Can you work these out from the model? Positions are in its coordinate system, mm. Give positions to 0.01 mm unless a question says otherwise; leave off trailing zeros. Loops run counter-clockwise (first coordinate to the right, second up) from the corner with the lowest first, then second, coordinate; pieces in that order, holes last.
Autodesk Inventor part; units mm, degrees
ref_plane "4DUMMY_XY" through (0, 0, 0) normal (1, 0, 0) x (0, 0, -1)
ref_plane "4DUMMY_YZ" through (0, 0, 0) normal (0, 0, -1) x (0, 1, 0)
ref_plane "4DUMMY_ZX" through (0, 0, 0) normal (0, 1, 0) x (1, 0, 0)
sketch "Sketch_15" plane through (-20, 0, 0) normal (1, 0, 0) x (0, 0, -1)
  line L0 (-7.5, 0.85) -> (-6.65, 0)
  line L1 (-6.65, 0) -> (6.65, 0)
  line L2 (6.65, 0) -> (7.5, 0.85)
  line L3 (7.5, 0.85) -> (7.5, 4.768)
  line L4 (7.5, 4.768) -> (5.4163, 5.9696)
  arc A0 (5.1599, 6.9262) -> (5.4163, 5.9696) centre (5.766, 6.576) ccw
  line L5 (5.1599, 6.9262) -> (6.6573, 9.518)
  arc A1 (7.5, 10.8638) -> (6.6573, 9.518) centre (8.107, 9.547) ccw
  line L6 (7.5, 10.8638) -> (7.5, 12.05)
  line L7 (7.5, 12.05) -> (7.05, 12.5)
  line L8 (7.05, 12.5) -> (6.6661, 12.5)
  arc A2 (4.8439, 12.5) -> (6.6661, 12.5) centre (5.755, 13.628) ccw
  line L9 (4.8439, 12.5) -> (-4.8439, 12.5)
  arc A3 (-6.6661, 12.5) -> (-4.8439, 12.5) centre (-5.755, 13.628) ccw
  line L10 (-6.6661, 12.5) -> (-7.05, 12.5)
  line L11 (-7.05, 12.5) -> (-7.5, 12.05)
  line L12 (-7.5, 12.05) -> (-7.5, 10.8638)
  arc A4 (-6.6573, 9.518) -> (-7.5, 10.8638) centre (-8.107, 9.547) ccw
  line L13 (-6.6573, 9.518) -> (-5.1599, 6.9262)
  arc A5 (-5.4163, 5.9696) -> (-5.1599, 6.9262) centre (-5.766, 6.576) ccw
  line L14 (-5.4163, 5.9696) -> (-7.5, 4.768)
  line L15 (-7.5, 4.768) -> (-7.5, 0.85)
extrude "Extrusion1" add sketch "Sketch_15" along normal blind 520
sketch "Sketch2" plane through (-20, 12.5, -4.8439) normal (0, 1, 0) x (1, 0, 0)
  point P0 (20, -4.8439)
hole "Hole1" at (0, 12.5, 0) direction (0, -1, 0) diameter 3.5 depth 12.5 counterbore diameter 6 counterbore depth 4.5
pattern_linear "Rectangular Pattern1" count 9 spacing 60 along (1, 0, 0) of "Hole1"
ref_plane "4DUMMY_XY" through (0, 0, 0) normal (1, 0, 0) x (0, 0, -1)
ref_plane "4DUMMY_YZ" through (0, 0, 0) normal (0, 0, -1) x (0, 1, 0)
ref_plane "4DUMMY_ZX" through (0, 0, 0) normal (0, 1, 0) x (1, 0, 0)
ref_plane "4SLIDE_XY" through (-20, 4.5, 0) normal (1, 0, 0) x (0, 0, -1)
ref_plane "4SLIDE_YZ" through (-20, 4.5, 0) normal (0, 0, -1) x (0, 1, 0)
ref_plane "4SLIDE_ZX" through (-20, 4.5, 0) normal (0, 1, 0) x (1, 0, 0)
ref_plane "4TRACK_XY" through (0, 0, 0) normal (0, 0, 1) x (1, 0, 0)
ref_plane "4TRACK_YZ" through (0, 0, 0) normal (1, 0, 0) x (0, 1, 0)
ref_plane "4TRACK_ZX" through (0, 0, 0) normal (0, 1, 0) x (0, 0, 1)
properties part number "SR15W52020 Track" material "Steel, Alloy"
(1) Please list where these lines run through material, in increasing order: probe 1 along Z at (x, y) = (240.5, 2.5); probe 2 along Z at (x, y) = (240, 10.55); probe 3 along Y at (x, z) = (351, 5.5).
Returned:
probe 1: z = -7.5 to -1.68, 1.68 to 7.5
probe 2: z = -7.06 to -3, 3 to 7.06
probe 3: y = 0 to 5.92, 7.51 to 12.2
(2) Suppose I cut it at A-A on x = 282. List the corners of the cut face in (y, z) for me (3 decimals).
Returned:
outline: (0, -6.65) - (0.85, -7.5) - (4.768, -7.5) - (5.97, -5.416) arc R0.7 cw to (6.926, -5.16) - (9.518, -6.657) arc R1.45 cw to (10.864, -7.5) - (12.05, -7.5) - (12.5, -7.05) - (12.5, -6.666) arc R1.45 cw to (12.5, -4.844) - (12.5, 4.844) arc R1.45 cw to (12.5, 6.666) - (12.5, 7.05) - (12.05, 7.5) - (10.864, 7.5) arc R1.45 cw to (9.518, 6.657) - (6.926, 5.16) arc R0.7 cw to (5.97, 5.416) - (4.768, 7.5) - (0.85, 7.5) - (0, 6.65) - close
(3) Will this pin go through, and if not, where does the flat tip stop? P1, Ø4.5, axis at x = 60, z = 0, coming from the +Y side.
Returned:
P1: stops at y = 8
